Autodesk Inventor part; units mm, degrees
ref_plane "YZ Plane" through (0, 0, 0) normal (1, 0, 0) x (0, 1, 0)
ref_plane "XZ Plane" through (0, 0, 0) normal (0, 1, 0) x (-1, 0, 0)
ref_plane "XY Plane" through (0, 0, 0) normal (0, 0, 1) x (1, 0, 0)
sketch "Sketch1" plane through (0, 0, 0) normal (0, 0, 1) x (1, 0, 0)
  line L0 (0, 0) -> (25, 0)
  line L1 (25, 0) -> (25, 600)
  line L2 (25, 600) -> (0, 600)
  line L3 (0, 600) -> (0, 0)
  dimension "d0" = 25
  dimension "d1" = 600
extrude "Extrusion1" add sketch "Sketch1" along normal blind 25
chamfer "Chamfer1" distance 5 angle 45 12 edges at (25, 300, 25) (25, 300, 0) (0, 300, 25) (0, 600, 12.5) (12.5, 600, 0) (12.5, 600, 25) (25, 600, 12.5) (25, 0, 12.5) (12.5, 0, 25) (12.5, 0, 0) (0, 0, 12.5) (0, 300, 0)
properties part number "frame"
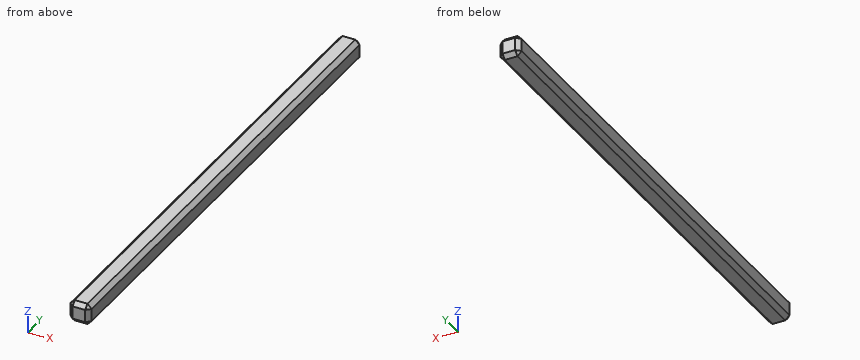
Build history of the part. All positions in model axes, mm. Round coordinates to 2 decimals unless told otherwise and drop trailing zeros. Order: outer loops, then holes, each group sorted by start corner. A loop starts at its lowest first (then second) coordinate and runs counter-clockwise, first axis right, second up. Notation, with made-up numbers: (10.5, -38) - (40.5, -38) arc R30 ccw to (40.5, -9) - close; hole circle Ø8 at (-26.5, -24). An arc over 180 degrees is marked (long way). Use a Markdown table: item, result.
1) Saw through at A-A on y = 522. Write the cut outline in (x, z).
Recorded:
| item | result |
|---|---|
| outline | (0, 5) - (5, 0) - (20, 0) - (25, 5) - (25, 20) - (20, 25) - (5, 25) - (0, 20) - close |
2) Wall check: L1, parallel to X at y = 226.5, z = 23.75; L2, parallel to Y at x = 2, z = 13; L3, parallel to X at y = 241, z = 23. Give the ranges that are in metal, low to high.
Recorded:
| item | result |
|---|---|
| L1 | x = 3.75 to 21.25 |
| L2 | y = 3 to 597 |
| L3 | x = 3 to 22 |
3) Flat gauge pins, fed straight in: pin 1 Ø2 at (x, z) = (3, 17.5) entering from -Y; pin 2 Ø6 at (x, z) = (22.5, 2.5) entering from +Y. Where does each tip first touch, or does it go through?
Recorded:
| item | result |
|---|---|
| pin 1 | stops at y = 1 |
| pin 2 | stops at y = 599.24 |
